Build history of the part. All positions in model axes, mm. A direction names the side the tool comes from. Give positions to 0.01 mm unless a question says otherwise; leave off trailing zeros. Order: outer loops, then holes, each group sorted by start corner. A loop starts at its lowest first (then second) coordinate and runs counter-clockwise, first axis right, second up. Notation, with made-up numbers: (36, -6.5) - (85, -6.5) arc R22 ccw to (85, 27.5) - close; hole circle Ø2 at (83.25, 49). An arc over 180 degrees is marked (long way). Use a Markdown table: item, result. Add a question column.
(1) Slice it at D-D (z = 3.5). Write the cut outline in (x, y).
(2) Mould opens along X. For faces 1 (the face through (7, -17, 15)), 2 (the face through (10.382, -19.961, 9.93)), 3 (the face through (14, -14, 14.25)) say: +X half, -X half, draft (parallel to the pull), parting line (faces both ways), or undercut.
(3) Wall check: line 1 (X direction, y = 11, z = 14.5); line 2 (Z direction, x = -14, y = -6); line 3 (X direction, y = -13.5, z = 11.5). Give the ranges that are in metal, low to high.
(4) Slice it at C-C (z = 6.75). Write the cut outline in (x, y), then the cut area to 3 significant figures.
(5) Flat gauge pins, fed straight in: pin 1 (1 mm diameter, centred on y = 4, z = 2, fed in from +X); pin 2 (0.6 mm diameter, centred on x = 0.5, y = -15.5, fed in from +Z); pin 3 (4 mm diameter, centred on y = 9, z = 7.5, fed in from +X). Where does each tip first touch, or does it go through?
(6) Which spindle directions (+Z, -Z, +X, -X, +Y, -Y) get a long thin tool onto all of the face, cutting with end or side? Do faces 4 (the face through (0, 0, 0)), 5 (the face through (-12.5, 0, 9)). Say none if no direction does.
from build123d import *

# Parameters (mm, degrees)
F0_R      = 22.5
F1_DEPTH  = 15
F2_R      = 18
F3_DEPTH  = 2.1
F4_W      = 25
F4_H      = 25
F5_DEPTH  = 8
F6_R      = 5
F7_R      = 1
F8_DEPTH  = 5
F9_R      = 20.5
F9_R_2    = 19
F10_DEPTH = 0.75


with BuildPart() as f1:
    # F0 (on Top) → F1 (new body)
    with BuildSketch(Plane.XY):
        Circle(F0_R)
    extrude(amount=F1_DEPTH)

    # F2 (on face) → F3 (cut)
    with BuildSketch(Plane.XY.offset(15)):
        Circle(F2_R)
    extrude(amount=-F3_DEPTH, mode=Mode.SUBTRACT)

    # F4 (on face) → F5 (cut)
    with BuildSketch(Plane.XY.offset(12.9)):
        Rectangle(F4_W, F4_H)
    extrude(amount=-F5_DEPTH, mode=Mode.SUBTRACT)

    # F6
    f6_edges = [f1.edges().sort_by_distance(p)[0] for p in [
        (-22.5, 0, 0),
    ]]
    fillet(f6_edges, radius=F6_R)

    # F7 (on face) → F8 (cut)
    with BuildSketch(Plane.XY.offset(12.9)):
        with Locations((0, 15.556349)):
            Circle(F7_R)
        with Locations((15.556349, 0)):
            Circle(F7_R)
        with Locations((-15.556349, 0)):
            Circle(F7_R)
        with Locations((0, -15.556349)):
            Circle(F7_R)
    extrude(amount=-F8_DEPTH, mode=Mode.SUBTRACT)

    # F9 (on face) → F10 (cut)
    with BuildSketch(Plane.XY.offset(15)):
        Circle(F9_R)
        Circle(F9_R_2, mode=Mode.SUBTRACT)
    extrude(amount=-F10_DEPTH, mode=Mode.SUBTRACT)


solid = f1.part
Solution:
| question | item | result |
|---|---|---|
| 1 | outline | circle Ø44.54 at (0, 0) |
| 2 | face 1 | draft |
| 2 | face 2 | parting line |
| 2 | face 3 | undercut |
| 3 | line 1 | -19.63 to -17.3, -15.49 to -14.25, 14.25 to 15.49, 17.3 to 19.63 |
| 3 | line 2 | 0 to 12.9 |
| 3 | line 3 | -18 to 18 |
| 4 | outline | circle Ø45 at (0, 0); hole (-12.5, -12.5) - (12.5, -12.5) - (12.5, 12.5) - (-12.5, 12.5) - close |
| 4 | area | 965 mm2 |
| 5 | pin 1 | x = 21.47 |
| 5 | pin 2 | z = 7.9 |
| 5 | pin 3 | x = 21.38 |
| 6 | face 4 | -Z, +X, -X, +Y, -Y |
| 6 | face 5 | +Z |
